```python
from build123d import *

# Parameters (mm, degrees)
SKETCH1_R                                          = 78.359
SKETCH1_R_2                                        = 37.5031
BOSS_EXTRUDE1_DEPTH                                = 7.62
CSK_FOR_10_FLAT_HEAD_MACHINE_SCREW_100_D           = 4.9784
CSK_FOR_10_FLAT_HEAD_MACHINE_SCREW_100_CSINK_D     = 9.779
CSK_FOR_10_FLAT_HEAD_MACHINE_SCREW_100_CSINK_ANGLE = 100
CIRPATTERN1_COUNT                                  = 3
SKETCH6_R                                          = 78.359
SKETCH6_R_2                                        = 76.1746
CUT_EXTRUDE1_DEPTH                                 = 2.54
FILLET1_R                                          = 1.5875


with BuildPart() as part:
    # Sketch1 → Boss-Extrude1 (new body)
    with BuildSketch(Plane(origin=(0, 0, 0), x_dir=(1, 0, 0), z_dir=(0, 1, 0))):
        with Locations(Location((0, 0, 0), (0, 0, 90))):
            Circle(SKETCH1_R)
        with Locations(Location((0, 0, 0), (0, 0, 90))):
            Circle(SKETCH1_R_2, mode=Mode.SUBTRACT)
    extrude(amount=BOSS_EXTRUDE1_DEPTH)

    # CSK for #10 Flat Head Machine Screw (100)1 (through all)
    with Locations(Plane(origin=(0, 7.62, 0), x_dir=(1, 0, 0), z_dir=(0, 1, 0))):
        with Locations((57.15, 0)):
            csk_for_10_flat_head_machine_screw_100 = CounterSinkHole(CSK_FOR_10_FLAT_HEAD_MACHINE_SCREW_100_D / 2, CSK_FOR_10_FLAT_HEAD_MACHINE_SCREW_100_CSINK_D / 2, counter_sink_angle=CSK_FOR_10_FLAT_HEAD_MACHINE_SCREW_100_CSINK_ANGLE)

    # CirPattern1: CSK for #10 Flat Head Machine Screw (100)1 ×3 about axis
    cirpattern1_axis = Axis((0, 0, 0), (0, 1, 0))
    for i in range(1, CIRPATTERN1_COUNT):
        add(csk_for_10_flat_head_machine_screw_100.rotate(cirpattern1_axis, i * 360 / CIRPATTERN1_COUNT), mode=Mode.SUBTRACT)

    # Sketch6 → Cut-Extrude1 (cut)
    with BuildSketch(Plane.XZ):
        with Locations(Location((0, 0, 0), (0, 0, 270))):
            Circle(SKETCH6_R)
        with Locations(Location((0, 0, 0), (0, 0, 270))):
            Circle(SKETCH6_R_2, mode=Mode.SUBTRACT)
    extrude(amount=-CUT_EXTRUDE1_DEPTH, mode=Mode.SUBTRACT)

    # Fillet1
    fillet1_edges = [part.edges().sort_by_distance(p)[0] for p in [
        (0, 2.54, 78.359),
        (0, 7.62, 78.359),
    ]]
    fillet(fillet1_edges, radius=FILLET1_R)


solid = part.part
```
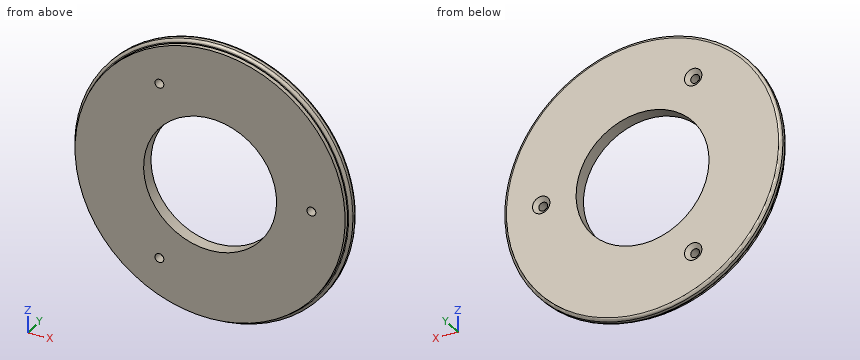
Could you check a few things on this model? Use its own coordinates, in mm. Give positions to 0.01 mm unless a question says otherwise; leave off trailing zeros. Loops run counter-clockwise (first coordinate to the right, second up) from the corner with the lowest first, then second, coordinate; pieces in that order, holes last. Notation, with made-up numbers: (-11, 71.5) - (-2, 71.5) arc R22 ccw to (-2, 80.5) - close; hole circle Ø1 at (-22, -5.75). An arc over 180 degrees is marked (long way). Answer in a Markdown table with one row per item. Add a question column.
Q1. If we section it at B-B (z = 0): List the corners of the cut face in (x, y) for me (1 decimal), plus the area to 3 significant figures.
Q2. Please list where these lines run through material, in increasing order: L1, parallel to Z at x = 7.5, y = 2.75; L2, parallel to Z at x = -23, y = 5.25; L3, parallel to X at y = 0.75, z = -13. Write a range as from..to.
Q3. If we section it at A-A (x = 0): List the corners of the cut face in (y, z) for me (1 decimal), plus the area to 3 significant figures.
Q4. For pin 1 (3 mm diameter, centred on x = -6.5, z = -39.5, fed in from -Y); pin 2 (5.5 mm diameter, centred on x = -28.57, z = -49.49, fed in from +Y); pin 3 (4 mm diameter, centred on y = 2.5, z = 41.5, fed in from -X); pin 4 (3 mm diameter, centred on y = 4.5, z = -13.5, fed in from -X), each with a flat end and sliding along its axis, tell me the tip position at first contact or that it passes through.
The answers:
| question | item | result |
|---|---|---|
| 1 | outline | (-78.4, 4.1) arc R1.6 ccw to (-76.8, 2.5) - (-76.2, 2.5) - (-76.2, 0) - (-37.5, 0) - (-37.5, 7.6) - (-76.8, 7.6) arc R1.6 ccw to (-78.4, 6) - close; (37.5, 0) - (54.7, 0) - (54.7, 5.6) - (52.3, 7.6) - (37.5, 7.6) - close; (59.6, 0) - (76.2, 0) - (76.2, 2.5) - (76.8, 2.5) arc R1.6 ccw to (78.4, 4.1) - (78.4, 6) arc R1.6 ccw to (76.8, 7.6) - (62, 7.6) - (59.6, 5.6) - close |
| 1 | area | 567 mm^2 |
| 2 | L1 | z = -77.2..-36.75, 36.75..77.2 |
| 2 | L2 | z = -74.91..-29.62, 29.62..74.91 |
| 2 | L3 | x = -75.06..-35.18, 35.18..75.06 |
| 3 | outline | (0, -76.2) - (2.5, -76.2) - (2.5, -76.8) arc R1.6 ccw to (4.1, -78.4) - (6, -78.4) arc R1.6 ccw to (7.6, -76.8) - (7.6, -37.5) - (0, -37.5) - close; (0, 37.5) - (7.6, 37.5) - (7.6, 76.8) arc R1.6 ccw to (6, 78.4) - (4.1, 78.4) arc R1.6 ccw to (2.5, 76.8) - (2.5, 76.2) - (0, 76.2) - close |
| 3 | area | 609 mm^2 |
| 4 | pin 1 | stops at y = 0 |
| 4 | pin 2 | stops at y = 5.83 |
| 4 | pin 3 | stops at x = -67.38 |
| 4 | pin 4 | stops at x = -77.43 |
